Design review of the part built by this model. Coordinates are the model's own, in mm. A direction names the side the tool comes from. Coordinates: 2 decimals unless noted, no trailing zeros. Loops run counter-clockwise (first coordinate to the right, second up) from the corner with the lowest first, then second, coordinate; pieces in that order, holes last.
Q1. Add section D-D on x = 62.5. Give the boundary of the cut face in (y, z).
Q2. Add section A-A on x = 0. Give the boundary of the cut face in (y, z), and give its area (3 significant figures).
Q3. Wall thickness on probe 1 along X at (y, z) = (6.25, 29.5); probe 2 along X at (y, z) = (9, 27); probe 3 along Z at (x, y) = (31, -1.5): over which ranges is each line inside the solid? List them lowest first.
Q4. Draft analysis for pull direction Z (two halves, no side actions). For faces 6 (the face through (-1, 12.7, 3)), 7 (the face through (-78.27, -0.18, 14.76)), 8 (the face through (97.061, 2.398, -29.177)), state which applies: released by +Z, released by -Z, zero draft, split by the parting line, or undercut.
Q5. For P1, Ø5, axis at x = -72.5, y = -6, coming from the +Z side; P2, Ø10, axis at x = -45, y = -6, coming from the -Z side; P3, Ø12, axis at x = 89, y = -5, coming from the +Z side; P4, Ø12.5, axis at x = 15, y = 3, coming from the -Z side, all flat-tipped, find the tip position at first contact; note any pin that passes through.
Q6. Machinability: for faces 1 (the face through (-61.779, -0.178, 60.757)), 2 (the face through (-13.034, -0.178, 57.716)), 3 (the face through (-90, 0, 24.154)), 4 (the face through (-38.61, -0.18, -27.55)), 5 (the face through (1, 0, 31.397)), which of the approach directions +Z, -Z, +X, -X, +Y, -Y give a long, thin tool a straight path to every point of the face, cutting with its end or side? Answer none if there is none.
Q7. Add section C-C on z = 39. Give the boundary of the cut face in (x, y), and give its area (3 significant figures).
```python
from build123d import *

# Parameters (mm, degrees)
F1_DEPTH = 12.7
F2_SIZE  = 5.08


with BuildPart() as f1:
    # F0 (on Front) → F1 (new body, symmetric)
    with BuildSketch(Plane.XZ):
        with BuildLine():
            Line((-78.86985, 24.153677), (-77.649682, 5.103677))
            Line((-77.649682, 5.103677), (-101.346, 5.103677))
            Line((-101.346, 5.103677), (-101.346, -28.678323))
            Line((-101.346, -28.678323), (-92.893675, -29.661545))
            Line((-92.893675, -29.661545), (-45.212, -29.661545))
            Line((-45.212, -29.661545), (-31.82804, -25.383405))
            Line((-31.82804, -25.383405), (31.82804, -25.383405))
            Line((31.82804, -25.383405), (45.212, -29.661545))
            Line((45.212, -29.661545), (92.893675, -29.661545))
            Line((92.893675, -29.661545), (101.346, -28.678323))
            Line((101.346, -28.678323), (101.346, 5.103677))
            Line((101.346, 5.103677), (77.649682, 5.103677))
            Line((77.649682, 5.103677), (78.86985, 24.153677))
            Line((78.86985, 24.153677), (101.346, 24.153677))
            Line((101.346, 24.153677), (101.346, 33.805677))
            ThreePointArc((101.346, 33.805677), (99.237568, 40.813436), (93.612348, 45.494363))
            Line((93.612348, 45.494363), (70.308838, 55.395677))
            ThreePointArc((70.308838, 55.395677), (61.88423, 60.664586), (55.500858, 68.27957))
            ThreePointArc((55.500858, 68.27957), (50.637881, 73.685788), (44.103503, 76.876033))
            Line((44.103503, 76.876033), (19.907397, 83.368455))
            Line((19.907397, 83.368455), (6.35, 32.77156))
            Line((6.35, 32.77156), (-6.35, 32.77156))
            Line((-6.35, 32.77156), (-19.907397, 83.368455))
            Line((-19.907397, 83.368455), (-44.103503, 76.876033))
            ThreePointArc((-44.103503, 76.876033), (-50.637881, 73.685788), (-55.500858, 68.27957))
            ThreePointArc((-55.500858, 68.27957), (-61.88423, 60.664586), (-70.308838, 55.395677))
            Line((-70.308838, 55.395677), (-93.612348, 45.494363))
            ThreePointArc((-93.612348, 45.494363), (-99.237568, 40.813436), (-101.346, 33.805677))
            Line((-101.346, 33.805677), (-101.346, 24.153677))
            Line((-101.346, 24.153677), (-78.86985, 24.153677))
        make_face()
        with BuildLine():
            Line((33.285186, 12.346792), (-30.214814, 12.346792))
            ThreePointArc((-30.214814, 12.346792), (-39.345917, 22.065697), (-29.81886, 31.396792))
            Line((-29.81886, 31.396792), (33.285186, 31.396792))
            ThreePointArc((33.285186, 31.396792), (42.810186, 21.871792), (33.285186, 12.346792))
        make_face(mode=Mode.SUBTRACT)
    extrude(amount=F1_DEPTH, both=True)

    # F2
    f2_edges = [f1.edges().sort_by_distance(p)[0] for p in [
        (-97.119838, -12.7, -29.169934),
        (97.119838, -12.7, -29.169934),
    ]]
    chamfer(f2_edges, length=F2_SIZE)


solid = f1.part
```
Entries:
1. outline: (-12.7, -28.08) - (-11.13, -29.66) - (12.7, -29.66) - (12.7, 60.14) - (-12.7, 60.14) - close
2. outline: (-12.7, -25.38) - (12.7, -25.38) - (12.7, 12.35) - (-12.7, 12.35) - close; (-12.7, 31.4) - (12.7, 31.4) - (12.7, 32.77) - (-12.7, 32.77) - close
2. area: 993 mm2
3. probe 1: x = -101.35 to -35.52, 38.99 to 101.35
3. probe 2: x = -101.35 to -37.85, 41.31 to 101.35
3. probe 3: z = -25.38 to 12.35, 31.4 to 80.39
4. face 6: zero draft
4. face 7: undercut
4. face 8: released by -Z
5. P1: stops at z = 55.53
5. P2: stops at z = -29.66
5. P3: stops at z = 50
5. P4: stops at z = -25.38
6. face 1: +Z, -X, +Y, -Y
6. face 2: +Z, +Y, -Y
6. face 3: -X, +Y, -Y
6. face 4: -Z, +Y, -Y
6. face 5: +Y, -Y
7. outline: (-100.24, -12.7) - (-8.02, -12.7) - (-8.02, 12.7) - (-100.24, 12.7) - close; (8.02, -12.7) - (100.24, -12.7) - (100.24, 12.7) - (8.02, 12.7) - close
7. area: 4,680 mm2
